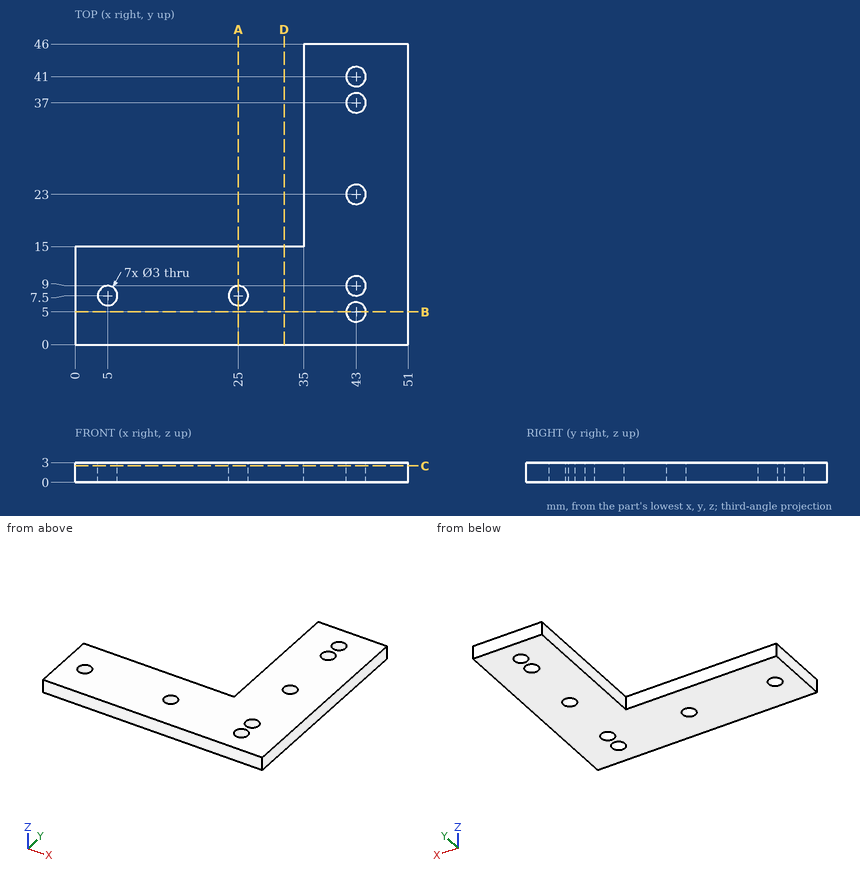
Job drawing, mm, ordinate dimensions from the low corner. One solid piece. Coordinates: 2 decimals unless noted, no trailing zeros. Write each loop counter-clockwise with the first axis right and the second up, starting at its lowest first coordinate (ties: lowest second). Pieces come first, ordered by that corner, then holes. Notation, with made-up numbers: (41, 40) - (67, 40) arc R23 cw to (67, 63) - close; hole circle Ø11 at (80, 6). An arc over 180 degrees is marked (long way). Use a Markdown table: item, result. Add a question column.
Item 1: Band-saw the part on B-B, the plane y = 5. Give the cut face in (x, z), and give its area (3 significant figures).
Item 2: Drill centre lines: L1, parallel to Y at x = 43, z = 1.35; L2, parallel to X at y = 5, z = 1.35; L3, parallel to Y at x = 25, z = 0.7. Where is each one in solid material? Low to high. Write a range as from..to.
Item 3: Band-saw the part on C-C, the plane z = 2.5. Give the cut face in (x, y), and give its area (3 significant figures).
Item 4: Band-saw the part on D-D, the plane x = 32. Give the cut face in (y, z).
Item 5: Band-saw the part on A-A, the plane x = 25. Give the cut face in (y, z).
Item 6: Flat gauge pin, fed straight in: pin 1 (0.9 mm diameter, centred on x = 19.5, z = 1.5, fed in from +Y). Where does the tip first touch, or does it go through?
Numbers:
| question | item | result |
|---|---|---|
| 1 | outline | (0, 0) - (41.5, 0) - (41.5, 3) - (0, 3) - close; (44.5, 0) - (51, 0) - (51, 3) - (44.5, 3) - close |
| 1 | area | 144 mm2 |
| 2 | L1 | 0..3.5, 6.5..7.5, 10.5..21.5, 24.5..35.5, 38.5..39.5, 42.5..46 |
| 2 | L2 | 0..41.5, 44.5..51 |
| 2 | L3 | 0..6, 9..15 |
| 3 | outline | (0, 0) - (51, 0) - (51, 46) - (35, 46) - (35, 15) - (0, 15) - close; hole circle Ø3 at (5, 7.5); hole circle Ø3 at (25, 7.5); hole circle Ø3 at (43, 5); hole circle Ø3 at (43, 9); hole circle Ø3 at (43, 23); hole circle Ø3 at (43, 37); hole circle Ø3 at (43, 41) |
| 3 | area | 1,210 mm2 |
| 4 | outline | (0, 0) - (15, 0) - (15, 3) - (0, 3) - close |
| 5 | outline | (0, 0) - (6, 0) - (6, 3) - (0, 3) - close; (9, 0) - (15, 0) - (15, 3) - (9, 3) - close |
| 6 | pin 1 | y = 15 |
